Source: CAD feature listing. Evaluate the final solid. Frame: model axes, mm. A direction names the side the tool comes from. Round coordinates to 2 decimals unless told otherwise and drop trailing zeros. Order: outer loops, then holes, each group sorted by start corner. A loop starts at its lowest first (then second) coordinate and runs counter-clockwise, first axis right, second up. Notation, with made-up numbers: (40.5, -18.75) -> (45.5, -18.75) arc R15 ccw to (45.5, 2.25) -> close; hole circle Ø6 at (25, 32). An arc over 180 degrees is marked (long way). One line per item, written item: value. Start each with the question number.
1) Reachability of faces 1 (the face through (-0.897, 0.282, -6.49)), 2 (the face through (-2.875, 0.99, -11.677)) from +Z, -Z, +X, -X, +Y, -Y: full face, straight path, thin tool, end or side. Return the list, or none.
2) Section D-D (y = 0). Return the cut outline in (x, z), and give its area (3 significant figures).
3) Mould query, pull axis X, two halves, no side actions, for faces 3 (the face through (-3.007, 0.009, -11.613)), 4 (the face through (0, 0, -12.8)), 5 (the face through (2.847, -0.997, -11.581)). Classes: pulls with the +X half, pulls with the -X half, needs draft (parallel to the pull), parting line crosses it, or undercut.
4) Section C-C (z = -7.5). Return the cut outline in (x, y).
5) Section A-A (x = 0). Return the cut outline in (y, z).
6) Pin query (flat end, axial travel): P1, Ø2, axis at x = 0, z = -19, coming from the +Y side; P2, Ø3.5, axis at x = 0, z = -17.5, coming from the -Y side; P3, Ø2, axis at x = -2.5, z = -4.5, coming from the +Y side. Return the tip coordinate at first contact, or that it passes through.
7) Ray query, L1, parallel to Y at x = 0, z = -8; L2, parallel to X at y = 0.55, z = -21.25. Return the intervals inside material, ascending.
8) Section B-B (z = -20.5). Return the cut outline in (x, y).
```python
from build123d import *

# Parameters (mm, degrees)
FLAT_DEPTH  = 1.14
FILLET2_R   = 0.5
FILLET2_2_R = 1


with BuildPart() as part:
    # Sketch1 → Revolve1 (revolve)
    with BuildSketch(Plane(origin=(0, 0, 0), x_dir=(1, 0, 0), z_dir=(0, 1, 0))):
        with BuildLine():
            Line((0, 12.8), (0, 16.8))
            ThreePointArc((0, 16.8), (-1.697056275, 16.097056275), (-2.4, 14.4))
            Line((-2.4, 14.4), (-2.4, 0))
            Line((-2.4, 0), (-0.94, 0))
            Line((-0.94, 0), (-0.94, 12.8))
            Line((-0.94, 12.8), (0, 12.8))
        make_face()
    revolve(axis=Axis((0, 0, -12.8), (0, 0, -1)))

    # Sketch3 → Flat (add, symmetric)
    with BuildSketch(Plane(origin=(0, 0, 0), x_dir=(1, 0, 0), z_dir=(0, 1, 0))):
        with BuildLine():
            Line((3.721476007, 14.971925444), (0.94, 1.886109672))
            Line((0.94, 1.886109672), (0.94, 12.8))
            Line((0.94, 12.8), (-0.94, 12.8))
            Line((-0.94, 12.8), (-0.94, 1.886109672))
            Line((-0.94, 1.886109672), (-3.721476007, 14.971925444))
            ThreePointArc((-3.721476007, 14.971925444), (-3.885218954, 16.00575772), (-3.94, 17.051042353))
            Line((-3.94, 17.051042353), (-3.94, 21.06))
            ThreePointArc((-3.94, 21.06), (0, 25), (3.94, 21.06))
            Line((3.94, 21.06), (3.94, 17.051042353))
            ThreePointArc((3.94, 17.051042353), (3.885218954, 16.00575772), (3.721476007, 14.971925444))
        make_face()
    extrude(amount=FLAT_DEPTH, both=True)

    # Fillet2
    fillet2_edges = [part.edges().sort_by_distance(p)[0] for p in [
        (0, 1.14, -25),
        (0, -1.14, -25),
    ]]
    fillet(fillet2_edges, radius=FILLET2_R)

    # Fillet2 2
    fillet2_2_edges = [part.edges().sort_by_distance(p)[0] for p in [
        (2.4, 0, 0),
    ]]
    fillet(fillet2_2_edges, radius=FILLET2_2_R)

    # Sketch4 → Ball Hole (revolve, cut)
    with BuildSketch(Plane(origin=(0, 0, 0), x_dir=(1, 0, 0), z_dir=(0, 1, 0))):
        with BuildLine():
            Line((0, 23.44), (0, 18.68))
            ThreePointArc((0, 18.68), (2.38, 21.06), (0, 23.44))
        make_face()
    revolve(axis=Axis((0, 0, -23.44), (0, 0, 1)), mode=Mode.SUBTRACT)


solid = part.part
```
Findings:
1. face 1: +Z
1. face 2: +Z, -X, +Y
2. outline: (-3.94, -21.06) arc R3.94 ccw to (3.94, -21.06) -> (3.94, -17.05) arc R10 ccw to (3.72, -14.97) -> (2.4, -8.75) -> (2.4, -1) arc R1 ccw to (1.4, 0) -> (0.94, 0) -> (0.94, -12.8) -> (-0.94, -12.8) -> (-0.94, 0) -> (-1.4, 0) arc R1 ccw to (-2.4, -1) -> (-2.4, -8.75) -> (-3.72, -14.97) arc R10 ccw to (-3.94, -17.05) -> close; hole circle Ø4.76 at (0, -21.06)
2. area: 110 mm2
3. face 3: pulls with the -X half
3. face 4: undercut
3. face 5: pulls with the +X half
4. outline: circle Ø4.8 at (0, 0); hole circle Ø1.88 at (0, 0)
5. outline: (-2.4, -14.4) arc R2.4 ccw to (-1.14, -16.51) -> (-1.14, -18.97) arc R2.38 cw to (1.14, -18.97) -> (1.14, -16.51) arc R2.4 ccw to (2.4, -14.4) -> (2.4, -1) arc R1 ccw to (1.4, 0) -> (0.94, 0) -> (0.94, -12.8) -> (-0.94, -12.8) -> (-0.94, 0) -> (-1.4, 0) arc R1 ccw to (-2.4, -1) -> close; (-1.14, -24.5) arc R0.5 ccw to (-0.64, -25) -> (0.64, -25) arc R0.5 ccw to (1.14, -24.5) -> (1.14, -23.15) arc R2.38 cw to (-1.14, -23.15) -> close
6. P1: y = 1.14
6. P2: y = -1.98
6. P3: y = 1.87
7. L1: -2.4 to -0.94, 0.94 to 2.4
7. L2: -3.94 to -2.31, 2.31 to 3.94
8. outline: (-3.94, -0.64) arc R0.5 ccw to (-3.44, -1.14) -> (-2.01, -1.14) arc R2.31 cw to (-2.01, 1.14) -> (-3.44, 1.14) arc R0.5 ccw to (-3.94, 0.64) -> close; (2.01, -1.14) -> (3.44, -1.14) arc R0.5 ccw to (3.94, -0.64) -> (3.94, 0.64) arc R0.5 ccw to (3.44, 1.14) -> (2.01, 1.14) arc R2.31 cw to start
